Can you work these out from the model? Positions are in its coordinate system, mm. A direction names the side the tool comes from. Round coordinates to 2 decimals unless told otherwise and drop trailing zeros. Loops run counter-clockwise (first coordinate to the right, second up) from the corner with the lowest first, then second, coordinate; pieces in that order, holes last. Notation, with made-up numbers: (31.5, -23) - (62.5, -23) arc R21 ccw to (62.5, 15) - close; hole circle Ø1 at (33, 41.25). An arc over 180 degrees is marked (long way). Answer as CSV lines item,"result".
```python
from build123d import *

# Parameters (mm, degrees)
SKETCH1_W           = 30
SKETCH1_H           = 30
BOSS_EXTRUDE1_DEPTH = 2
SKETCH2_R           = 1
CUT_EXTRUDE1_DEPTH  = 2
SKETCH3_W           = 4
SKETCH3_H           = 30
BOSS_EXTRUDE2_DEPTH = 25
CUT_EXTRUDE2_DEPTH  = 38
BOSS_EXTRUDE3_DEPTH = 7
CUT_EXTRUDE3_DEPTH  = 7


with BuildPart() as part:
    # Sketch1 → Boss-Extrude1 (new body)
    with BuildSketch(Plane(origin=(0, 0, 0), x_dir=(1, 0, 0), z_dir=(0, 1, 0))):
        Rectangle(SKETCH1_W, SKETCH1_H)
    extrude(amount=BOSS_EXTRUDE1_DEPTH)

    # Sketch2 → Cut-Extrude1 (cut)
    with BuildSketch(Plane(origin=(0, 2, 0), x_dir=(1, 0, 0), z_dir=(0, 1, 0))):
        with Locations(Location((0, 8, 0), (0, 0, 270))):
            Circle(SKETCH2_R)
        with Locations(Location((8, 0, 0), (0, 0, 270))):
            Circle(SKETCH2_R)
        with Locations(Location((0, -8, 0), (0, 0, 270))):
            Circle(SKETCH2_R)
        with Locations(Location((-8, 0, 0), (0, 0, 270))):
            Circle(SKETCH2_R)
    extrude(amount=-CUT_EXTRUDE1_DEPTH, mode=Mode.SUBTRACT)

    # Sketch3 → Boss-Extrude2 (add)
    with BuildSketch(Plane(origin=(0, 2, 0), x_dir=(1, 0, 0), z_dir=(0, 1, 0))):
        with Locations((-13, 0)):
            Rectangle(SKETCH3_W, SKETCH3_H)
        with Locations((13, 0)):
            Rectangle(SKETCH3_W, SKETCH3_H)
    extrude(amount=BOSS_EXTRUDE2_DEPTH)

    # Sketch5 → Cut-Extrude2 (cut)
    with BuildSketch(Plane.ZY.offset(15)):
        with BuildLine():
            Line((15, 27), (0, 27))
            ThreePointArc((0, 27), (3.892908452, 25.817668243), (6.470757107, 22.670075367))
            Line((6.470757107, 22.670075367), (15, 2))
            Line((15, 2), (15, 27))
        make_face()
        with BuildLine():
            ThreePointArc((-6.470757107, 22.670075367), (-3.892908452, 25.817668243), (0, 27))
            Line((0, 27), (-15, 27))
            Line((-15, 27), (-15, 2))
            Line((-15, 2), (-6.470757107, 22.670075367))
        make_face()
    extrude(amount=-CUT_EXTRUDE2_DEPTH, mode=Mode.SUBTRACT)

    # Sketch6 → Boss-Extrude3 (add)
    with BuildSketch(Plane.ZY.offset(-11)):
        Polygon((0, 25), (-4.330127019, 22.5), (-4.330127019, 17.5), (0, 15), (4.330127019, 17.5), (4.330127019, 22.5), align=None)
    extrude(amount=BOSS_EXTRUDE3_DEPTH)

    # Sketch7 → Cut-Extrude3 (cut)
    with BuildSketch(Plane.ZY.offset(15)):
        Polygon((0, 25), (-4.330127019, 22.5), (-4.330127019, 17.5), (0, 15), (4.330127019, 17.5), (4.330127019, 22.5), align=None)
    extrude(amount=-CUT_EXTRUDE3_DEPTH, mode=Mode.SUBTRACT)


solid = part.part
```
Q1. I'm going to push flat-ended pins straight in: pin 1 Ø1.6 at (x, z) = (8, 0) entering from +Y; pin 2 Ø8 at (x, y) = (-1, 24) entering from +Z; pin 3 Ø2 at (x, z) = (-4.5, 5) entering from +Y; pin 4 Ø4.5 at (x, y) = (-13.5, 21) entering from -Z. Where does each tip first touch, or does it pass through?
Checks:
pin 1,"y = 25"
pin 2,"through"
pin 3,"y = 2"
pin 4,"z = -8.09"
Q2. On a 3-axis mill with a long thin cutter (end or side, diameter ignored), from which of +Z, -Z, +X, -X, +Y, -Y can I reach the whole of each face in a straight line? I mean faces 1 (the flat face through (-13.03, 23.77, -2.13)), 2 (the cylindrical face through (9, 1, 0)), 3 (the flat face through (7.55, 16.23, 2.13)), 4 (the flat face through (8, 20, 4.33)), 5 (the flat face through (7.55, 23.77, -2.13)). Say none if no direction works.
Checks:
face 1,"-X"
face 2,"-Y"
face 3,"+Z"
face 4,"+Z, +Y"
face 5,"-Z, +Y"
Q3. If I drill on line 1 along X through (y, z) = (0.55, 0); line 2 along X through (y, z) = (13.5, 1.5); line 3 along X through (y, z) = (0.45, 8), over which ranges is the centre line in solid material (lowest first)? Write a range as [from, to].
Checks:
line 1,"[-15, -9], [-7, 7], [9, 15]"
line 2,"[-15, -11], [11, 15]"
line 3,"[-15, -1], [1, 15]"
Q4. Imagine slicing it at A-A (x = 8). Write out the boundary of the cut face in (y, z), then the cut area to 3 significant figures.
Checks:
outline,"(0, -15) - (2, -15) - (2, -1) - (0, -1) - close; (0, 1) - (2, 1) - (2, 15) - (0, 15) - close; (15, 0) - (17.5, -4.33) - (22.5, -4.33) - (25, 0) - (22.5, 4.33) - (17.5, 4.33) - close"
area,"121 mm²"
Q5. Imagine slicing it at D-D (x = -8). Write out the boundary of the cut face in (y, z).
Checks:
outline,"(0, -15) - (2, -15) - (2, -1) - (0, -1) - close; (0, 1) - (2, 1) - (2, 15) - (0, 15) - close"
Q6. Imagine slicing it at C-C (y = 4). Write out the boundary of the cut face in (x, z).
Checks:
outline,"(-15, -14.17) - (-11, -14.17) - (-11, 14.17) - (-15, 14.17) - close; (11, -14.17) - (15, -14.17) - (15, 14.17) - (11, 14.17) - close"
Q7. We'd pull the mould along Y, two halves only. Please class faces 6 (the cylindrical face through (-7, 1, 0)), 7 (the flat face through (-13, 20, 4.33)), 8 (the flat face through (12.972, 12.48, 10.676)): pulls with the +Y half, pulls with the -Y half, needs draft (parallel to the pull), parting line crosses it, or undercut.
Checks:
face 6,"needs draft"
face 7,"undercut"
face 8,"pulls with the +Y half"
Q8. Imagine slicing it at B-B (z = -8). Write out the boundary of the cut face in (x, y), then the cut area to 3 significant figures.
Checks:
outline,"(-15, 0) - (-1, 0) - (-1, 2) - (-11, 2) - (-11, 18.96) - (-15, 18.96) - close; (1, 0) - (15, 0) - (15, 18.96) - (11, 18.96) - (11, 2) - (1, 2) - close"
area,"192 mm²"
